Part model, mm, in its own coordinate system. A direction names the side the tool comes from. Give positions to 0.01 mm unless a question says otherwise; leave off trailing zeros. Write each loop counter-clockwise with the first axis right and the second up, starting at its lowest first coordinate (ties: lowest second). Pieces come first, ordered by that corner, then holes.
from build123d import *

# Parameters (mm, degrees)
SKETCH2_R           = 6
BOSS_EXTRUDE1_DEPTH = 6
SKETCH3_R           = 3
BOSS_EXTRUDE2_DEPTH = 15
CUT_EXTRUDE1_DEPTH  = 13
CUT_EXTRUDE2_DEPTH  = 0.5
SKETCH6_R           = 1.5
CUT_EXTRUDE3_DEPTH  = 2
CIRPATTERN1_COUNT   = 6
BOSS_EXTRUDE3_DEPTH = 6
SKETCH8_R           = 16
BOSS_EXTRUDE4_DEPTH = 2
SKETCH9_R           = 7
BOSS_EXTRUDE5_DEPTH = 6
SKETCH10_R          = 7
SKETCH10_R_2        = 1
CUT_EXTRUDE4_DEPTH  = 1
FILLET2_R           = 0.1
FILLET3_R           = 0.1
SKETCH11_W          = 6
SKETCH11_H          = 14
BOSS_EXTRUDE6_DEPTH = 5
SKETCH13_W          = 4
SKETCH13_H          = 13
CUT_EXTRUDE6_DEPTH  = 5
SKETCH14_W          = 5.026606417
SKETCH14_H          = 8
CUT_EXTRUDE7_DEPTH  = 1


with BuildPart() as part:
    # Sketch1 → Revolve1 (revolve)
    with BuildSketch(Plane(origin=(0, 0, 0), x_dir=(1, 0, 0), z_dir=(0, 1, 0))):
        with BuildLine():
            Line((0, 18.5), (-21, 18.5))
            Line((-21, 18.5), (-21, 0))
            Line((-21, 0), (32.9, 0))
            Line((32.9, 0), (32.9, 0.3))
            ThreePointArc((32.9, 0.3), (32.694974747, 0.794974747), (32.2, 1))
            Line((32.2, 1), (22.9, 1))
            Line((22.9, 1), (22.9, 15.1))
            ThreePointArc((22.9, 15.1), (22.636396103, 15.736396103), (22, 16))
            Line((22, 16), (0, 16))
            Line((0, 16), (0, 18.5))
        make_face()
    revolve(axis=Axis((-21, 0, 0), (1, 0, 0)))

    # Sketch2 → Boss-Extrude1 (add)
    with BuildSketch(Plane.ZY.offset(21)):
        with Locations((0, 6)):
            Circle(SKETCH2_R)
    extrude(amount=BOSS_EXTRUDE1_DEPTH)

    # Sketch3 → Boss-Extrude2 (add)
    with BuildSketch(Plane.ZY.offset(27)):
        with Locations((0, 6)):
            Circle(SKETCH3_R)
    extrude(amount=BOSS_EXTRUDE2_DEPTH)

    # Sketch4 → Cut-Extrude1 (cut)
    with BuildSketch(Plane.ZY.offset(42)):
        with BuildLine():
            Line((-1.658312395, 8.5), (1.658312395, 8.5))
            ThreePointArc((1.658312395, 8.5), (0, 9), (-1.658312395, 8.5))
        make_face()
    extrude(amount=-CUT_EXTRUDE1_DEPTH, mode=Mode.SUBTRACT)

    # Sketch5 → Cut-Extrude2 (cut)
    with BuildSketch(Plane.ZY.offset(21)):
        with BuildLine():
            ThreePointArc((-4.982608643, 10.916666667), (0, -1), (4.982608643, 10.916666667))
            ThreePointArc((4.982608643, 10.916666667), (0, -12), (-4.982608643, 10.916666667))
        make_face()
    extrude(amount=-CUT_EXTRUDE2_DEPTH, mode=Mode.SUBTRACT)

    # Sketch6 → Cut-Extrude3 (cut)
    with BuildSketch(Plane.ZY.offset(21)):
        with Locations((15, 0)):
            Circle(SKETCH6_R)
    cut_extrude3 = extrude(amount=-CUT_EXTRUDE3_DEPTH, mode=Mode.SUBTRACT)

    # CirPattern1: Cut-Extrude3 ×6 about axis
    cirpattern1_axis = Axis((0, 0, 0), (1, 0, 0))
    for i in range(1, CIRPATTERN1_COUNT):
        add(cut_extrude3.rotate(cirpattern1_axis, i * 360 / CIRPATTERN1_COUNT), mode=Mode.SUBTRACT)

    # Sketch7 → Boss-Extrude3 (add)
    with BuildSketch(Plane(origin=(22.9, 0, 0), x_dir=(0, 0, -1), z_dir=(1, 0, 0))):
        with BuildLine():
            Line((1.5, 11.410824506), (-1.5, 11.410824506))
            ThreePointArc((-1.5, 11.410824506), (-2.089175494, 12), (-1.5, 12.589175494))
            Line((-1.5, 12.589175494), (1.5, 12.589175494))
            ThreePointArc((1.5, 12.589175494), (2.089175494, 12), (1.5, 11.410824506))
        make_face()
        with BuildLine():
            Line((1.5, -11.410824506), (-1.5, -11.410824506))
            ThreePointArc((-1.5, -11.410824506), (-2.089175494, -12), (-1.5, -12.589175494))
            Line((-1.5, -12.589175494), (1.5, -12.589175494))
            ThreePointArc((1.5, -12.589175494), (2.089175494, -12), (1.5, -11.410824506))
        make_face()
    extrude(amount=BOSS_EXTRUDE3_DEPTH)

    # Sketch8 → Boss-Extrude4 (add)
    with BuildSketch(Plane(origin=(22.9, 0, 0), x_dir=(0, 0, -1), z_dir=(1, 0, 0))):
        Circle(SKETCH8_R)
    extrude(amount=BOSS_EXTRUDE4_DEPTH)

    # Sketch9 → Boss-Extrude5 (add)
    with BuildSketch(Plane(origin=(24.9, 0, 0), x_dir=(0, 0, -1), z_dir=(1, 0, 0))):
        Circle(SKETCH9_R)
    extrude(amount=BOSS_EXTRUDE5_DEPTH)

    # Sketch10 → Cut-Extrude4 (cut)
    with BuildSketch(Plane(origin=(24.9, 0, 0), x_dir=(0, 0, -1), z_dir=(1, 0, 0))):
        Circle(SKETCH10_R)
        Circle(SKETCH10_R_2, mode=Mode.SUBTRACT)
    extrude(amount=CUT_EXTRUDE4_DEPTH, mode=Mode.SUBTRACT)

    # Fillet2
    fillet2_edges = [part.edges().sort_by_distance(p)[0] for p in [
        (30.9, 0, 7),
    ]]
    fillet(fillet2_edges, radius=FILLET2_R)

    # Fillet3
    fillet3_edges = [part.edges().sort_by_distance(p)[0] for p in [
        (25.9, 0, 7),
    ]]
    fillet(fillet3_edges, radius=FILLET3_R)

    # Sketch11 → Boss-Extrude6 (add)
    with BuildSketch(Plane(origin=(24.9, 0, 0), x_dir=(0, 0, -1), z_dir=(1, 0, 0))):
        with Locations((13, 0)):
            Rectangle(SKETCH11_W, SKETCH11_H)
    boss_extrude6 = extrude(amount=BOSS_EXTRUDE6_DEPTH)

    # Sketch13 → Cut-Extrude6 (cut)
    with BuildSketch(Plane(origin=(0, 0, -16), x_dir=(-1, 0, 0), z_dir=(0, 0, -1))):
        with Locations((-27.4, 0)):
            Rectangle(SKETCH13_W, SKETCH13_H)
    cut_extrude6 = extrude(amount=-CUT_EXTRUDE6_DEPTH, mode=Mode.SUBTRACT)

    # Sketch14 → Cut-Extrude7 (cut)
    with BuildSketch(Plane(origin=(29.9, 0, 0), x_dir=(0, 0, -1), z_dir=(1, 0, 0))):
        with Locations((13.486696792, 0)):
            Rectangle(SKETCH14_W, SKETCH14_H)
    cut_extrude7 = extrude(amount=-CUT_EXTRUDE7_DEPTH, mode=Mode.SUBTRACT)

    # Mirror1: Boss-Extrude6, Cut-Extrude6, Cut-Extrude7 across plane
    add(boss_extrude6.mirror(Plane.XY))
    add(cut_extrude6.mirror(Plane.XY), mode=Mode.SUBTRACT)
    add(cut_extrude7.mirror(Plane.XY), mode=Mode.SUBTRACT)


solid = part.part
1) Flat gauge pins, fed straight in: P1, Ø6, axis at x = 7.5, z = 2, coming from the +Y side; P2, Ø3, axis at x = 28, z = -14, coming from the -Y side; P3, Ø3, axis at y = 10.5, z = 7.5, coming from the +X side. Where does each tip first touch, or does it go through?
Check result:
P1: stops at y = 16
P2: stops at y = -7
P3: stops at x = 24.9
2) Mould opens along Y. For faces 5 (the cylindrical face through (-34.39, 3.07, -0.65)), 6 (the flat face through (25.2, 0, 16)), 7 (the cylindrical face through (28.366, -2.681, -6.466)) say: +Y half, -Y half, draft (parallel to the pull), parting line (faces both ways), or undercut.
Check result:
face 5: parting line
face 6: draft
face 7: undercut
3) Drill centre lines: L1, parallel to Y at x = -20.75, z = 0; L2, parallel to X at y = 1, z = 4.5; L3, parallel to X at y = 4, z = 4. Where is each one in solid material? Low to high.
Check result:
L1: y = -18.5 to -12, -1 to 18.5
L2: x = -21 to 24.9, 25.9 to 30.9
L3: x = -27 to 24.9, 25.9 to 30.9
4) Saw through at A-A (x = -35). Write the cut outline in (y, z).
Check result:
outline: (8.5, -1.66) - (8.5, 1.66) arc R3 ccw (long way) to start
5) Saw through at B-B (x = 11). Write the cut outline in (y, z), and give its area (3 significant figures).
Check result:
outline: circle Ø32 at (0, 0)
area: 804 mm2
6) Saw through at C-C (x = -4). Write the cut outline in (y, z).
Check result:
outline: circle Ø37 at (0, 0)
7) 3-axis set-ups, long thin cutter, end or side, ignore diameter. For faces 1 (the flat face through (24.9, -5.3, 15.5)), 2 (the flat face through (29.4, 5, -14)), 3 (the cylindrical face through (32, -1, 0)), 4 (the flat face through (25.2, 0, -16)): which of +Z, -Z, +X, -X, +Y, -Y reach the whole face in a straight line?
Check result:
face 1: +Z, -Y
face 2: -Z
face 3: +X
face 4: -Z, +X, +Y, -Y
